from build123d import *

# Parameters (mm, degrees)
CORTE_EXTRUS_O1_DEPTH = 32.287217837
PADR_OCIRCULAR2_COUNT = 9
ESBO_O6_R             = 4
CORTE_EXTRUS_O2_DEPTH = 32.134624111
ESBO_O7_W             = 0.2
ESBO_O7_H             = 30
CORTE_EXTRUS_O3_DEPTH = 10


with BuildPart() as part:
    # Esboço2 → Revolução1 (revolve)
    with BuildSketch(Plane.XY, mode=Mode.PRIVATE) as revolu_o1_sk:
        with BuildLine():
            Line((0, 0), (0, 16.464198342))
            ThreePointArc((0, 16.464198342), (0.321571182, 19.304004673), (1.27, 22))
            Line((1.27, 22), (2.03, 22))
            ThreePointArc((2.03, 22), (2.978428818, 19.304004673), (3.3, 16.464198342))
            Line((3.3, 16.464198342), (3.3, 0))
            Line((3.3, 0), (0, 0))
        make_face()
    revolve(revolu_o1_sk.sketch.rotate(Axis((0, 0, 0), (1, 0, 0)), 90), axis=Axis((0, 0, 0), (1, 0, 0)))

    # Esboço5 → Corte-extrusão1 (cut, through all)
    with BuildSketch(Plane(origin=(0, 0, 0), x_dir=(0, 0, -1), z_dir=(1, 0, 0))):
        with BuildLine():
            ThreePointArc((3.547062102, 16.950885739), (5.413227359, 19.685368366), (8.05493296, 21.680702805))
            ThreePointArc((8.05493296, 21.680702805), (0, 23.128657961), (-8.05493296, 21.680702805))
            ThreePointArc((-8.05493296, 21.680702805), (-5.413227359, 19.685368366), (-3.547062102, 16.950885739))
            ThreePointArc((-3.547062102, 16.950885739), (0, 14.691157961), (3.547062102, 16.950885739))
        make_face()
    corte_extrus_o1 = extrude(amount=CORTE_EXTRUS_O1_DEPTH, mode=Mode.SUBTRACT)

    # PadrãoCircular2: Corte-extrusão1 ×9 about axis
    padr_ocircular2_axis = Axis((0, 0, 0), (1, 0, 0))
    for i in range(1, PADR_OCIRCULAR2_COUNT):
        add(corte_extrus_o1.rotate(padr_ocircular2_axis, i * 360 / PADR_OCIRCULAR2_COUNT), mode=Mode.SUBTRACT)

    # Esboço6 → Corte-extrusão2 (cut, through all)
    with BuildSketch(Plane(origin=(3.3, 0, 0), x_dir=(0, 0, -1), z_dir=(1, 0, 0))):
        Circle(ESBO_O6_R)
    extrude(amount=-CORTE_EXTRUS_O2_DEPTH, mode=Mode.SUBTRACT)

    # Esboço7 → Corte-extrusão3 (cut)
    with BuildSketch(Plane(origin=(3.3, 0, 0), x_dir=(0, 0, -1), z_dir=(1, 0, 0))):
        with Locations((0, 15)):
            Rectangle(ESBO_O7_W, ESBO_O7_H)
    extrude(amount=-CORTE_EXTRUS_O3_DEPTH, mode=Mode.SUBTRACT)


solid = part.part
Geometry: final body of the model. Coordinates: model frame, mm. A direction names the side the tool comes from. Give positions to 0.01 mm unless a question says otherwise; leave off trailing zeros. Write each loop counter-clockwise with the first axis right and the second up, starting at its lowest first coordinate (ties: lowest second). Pieces come first, ordered by that corner, then holes.
(1) Ray query, line 1 (Z direction, x = 2.05, y = 0); line 2 (Y direction, x = 1.5, z = 0); line 3 (Z direction, x = 0.7, y = 15). Return the intervals inside material, ascending.
(2) Cut plane A-A, the plane y = 5. Return loops of the section in (x, z), then the cut area to 3 significant figures.
(3) Mould query, pull axis Z, two halves, no side actions, for faces 5 (the cylindrical face through (1.63, 2.61, -14.46)), 6 (the cylindrical face through (1.6, -16, 10.7)), 7 (the cylindrical face through (1.63, 2.49, 14.48)), 8 (the cylindrical face through (1.6, -16, -10.7)). Classes: released by +Z, released by -Z, zero draft, split by the parting line, or undercut.
(4) Access query for faces 1 (the cylindrical face through (1.63, 11.38, 15.55)), 2 (the cylindrical face through (1.627, 7.725, 17.583)), 3 (the cylindrical face through (1.63, -1.25, -19.17)), 4 (the flat face through (0, 3, -3)). Directions: +Z, -Z, +X, -X, +Y, -Y. A direction counts if a zero-diameter tool reaches every point of the face in a straight line with its end or side. Return the directions, or none.
(5) Cut plane B-B, the plane y = -6. Return loops of the section in (x, z), then the cut area to 3 significant figures.
(6) First-contact query: P1, Ø1.6, axis at x = 1.5, y = 7, coming from the +Z side; P2, Ø1.5, axis at x = 1.5, z = 0, coming from the +Y side; P3, Ø1, axis at x = 0.5, y = 13, coming from the -Z side. Flat tips, straight axial feed; report the tip coordinate or a pass-through.
Values follow:
1. line 1: z = -16.11 to -4, 4 to 16.11
1. line 2: y = -22 to -4
1. line 3: z = -8.12 to -1.52, 1.52 to 8.12
2. outline: (0, -14.83) - (3.3, -14.83) - (3.3, -0.1) - (0, -0.1) - close; (0, 0.1) - (3.3, 0.1) - (3.3, 14.83) - (0, 14.83) - close
2. area: 97.2 mm2
3. face 5: released by -Z
3. face 6: undercut
3. face 7: released by +Z
3. face 8: undercut
4. face 1: +X, -X, +Y
4. face 2: +Z, +X, -X
4. face 3: -Z, +X, -X
4. face 4: +Z, -Z, -X, +Y, -Y
5. outline: (0, -14.01) - (3.3, -14.01) - (3.3, 14.01) - (0, 14.01) - close
5. area: 92.5 mm2
6. P1: stops at z = 17.65
6. P2: stops at y = 14.76
6. P3: stops at z = -8.46
